Autodesk Inventor part; units mm, degrees
ref_plane "Plan de construction1" through (50, 0, -25) normal (0, 0, 1) x (1, 0, 0)
ref_plane "Plan de construction2" through (50, 0, 35) normal (0, 0, -1) x (-1, 0, 0)
ref_plane "YZ Plane" through (0, 0, 0) normal (1, 0, 0) x (0, 1, 0)
sketch "Esquisse1" plane through (0, 0, 0) normal (0, 1, 0) x (-1, 0, 0)
  line L0 (0, 0) -> (-100, 0)
  line L1 (-100, 0) -> (-100, -25)
  line L2 (-100, -25) -> (0, -25)
  line L3 (0, -25) -> (0, 0)
  arc A0 (0, -25) -> (25, 0) centre (0, 0) ccw
  line L4 (25, 0) -> (0, 0)
  line L5 (0, 0) -> (0, -25)
  line L6 (-100, 0) -> (-100, -25)
  arc A1 (-125, 0) -> (-100, -25) centre (-100, 0) ccw
  line L7 (-100, 0) -> (-125, 0)
  dimension "d1" = 25
  dimension "d2" = 100
revolve "Révolution1" add sketch "Esquisse1" angle 360 about axis through (0, 0, 0) along (1, 0, 0)
ref_plane "Plan de construction1" through (50, 0, -25) normal (0, 0, 1) x (1, 0, 0)
sketch "Esquisse2" plane through (50, 0, -25) normal (0, 0, 1) x (1, 0, 0)
  arc A0 (-50, 25) -> (-50, -25) centre (-50, 0) ccw
  line L0 (-50, 0) -> (-71.6506, -12.5)
  line L1 (-71.6506, -12.5) -> (-84.1506, 9.1506)
  line L2 (-84.1506, 9.1506) -> (-62.5, 21.6506)
  line L3 (-62.5, 21.6506) -> (-50, 0)
  line L4 (-50, 0) -> (-31.3481, 0) construction
  line L5 (-50, 0) -> (-62.5, 21.6506)
  line L6 (-62.5, 21.6506) -> (-19.1987, 46.6506)
  line L7 (-19.1987, 46.6506) -> (-6.6987, 25)
  line L8 (-6.6987, 25) -> (-50, 0)
  line L9 (-50, -25) -> (-50, 25) construction
  line L10 (-50, 25) -> (75, 25) construction
  line L11 (-50, 25) -> (50, 25) construction
  dimension "d9" = 120
extrude "Extrusion1" cut sketch "Esquisse2" along normal blind 30
ref_plane "Plan de construction2" through (50, 0, 35) normal (0, 0, -1) x (-1, 0, 0)
sketch "Esquisse3" plane through (50, 0, 35) normal (0, 0, -1) x (-1, 0, 0)
  line L0 (50, 0) -> (71.2132, -12.2474) construction
  line L1 (71.2132, -12.2474) -> (50, 0) construction
  line L2 (50, 0) -> (50, 0) construction
  line L3 (65.2228, 7.3769) -> (52.2324, 14.8769) construction
  circle A0 centre (65.2228, 7.3769) radius 1.7
  circle A1 centre (52.2324, 14.8769) radius 1.7
  line L4 (71.2132, -12.2474) -> (93.5005, 26.3552) construction
  line L5 (52.2324, 14.8769) -> (45.2324, 2.7526) construction
  line L6 (6.6987, 25) -> (-50, 25) construction
  dimension "d12" = 14
  dimension "d22" = 3.4
  dimension "d23" = 3.4
  dimension "d30" = 15
  dimension "d31" = 30
extrude "Extrusion2" cut sketch "Esquisse3" along normal blind 30
sketch "Esquisse4" plane through (50, 0, 35) normal (0, 0, -1) x (-1, 0, 0)
  circle A0 centre (65.2228, 7.3769) radius 1.7
  circle A1 centre (65.2228, 7.3769) radius 3.25
  circle A2 centre (52.2324, 14.8769) radius 1.7
  circle A3 centre (52.2324, 14.8769) radius 3.25
  point P0 (50, 0)
  dimension "d26" = 6.5
  dimension "d27" = 6.5
extrude "Extrusion3" cut sketch "Esquisse4" along normal blind 20
equation "\"d23\" = d22"
equation "\"d27\" = d26"
properties part number "P1704_003_mainGauche"
Check sheet for the modelled part. Datum: model origin and axes. Units: mm. A direction names the side the tool comes from. Round coordinates to 2 decimals unless told otherwise and drop trailing zeros. Loops run counter-clockwise (first coordinate to the right, second up) from the corner with the lowest first, then second, coordinate; pieces in that order, holes last. Notation, with made-up numbers: (-40, 48) - (-30, 48) arc R4 ccw to (-30, 52) - close; hole circle Ø10 at (65, 52.25). An arc over 180 degrees is marked (long way). Write item = value, one per line. Start each with the question number.
Q1. Section check A-A (x = 97). Record the boundary of the cut face in (y, z), plus the area to 3 significant figures.
Q2. Thickness scan on L1, parallel to Y at x = 0.5, z = 6; L2, parallel to X at y = 0, z = 7; L3, parallel to Z at x = 103.5, y = -13.5. Record the ranges inside material, lowest first.
Q3. Section check B-B (y = -7.5). Record the boundary of the cut face in (x, z).
Q4. Section check C-C (z = 0). Record the boundary of the cut face in (x, y).
Q5. Release check for a two-part mould opening along X. For faces 1 (the face through (1, 10, 5)), 2 (the face through (-16.793, 8.028, 10.07)) record: pulls with the +X half, pulls with the -X half, needs draft (parallel to the pull), parting line crosses it, or undercut.
Q6. Section check D-D (z = -12). Record the boundary of the cut face in (x, y).
Q7. Depth check by flat-ended pin: P1, Ø2, axis at x = -15.22, y = 7.38, coming from the -Z side; P2, Ø5, axis at x = -2.23, y = 14.88, coming from the -Z side; P3, Ø1, axis at x = 67.5, z = -19, coming from the +Y side; P4, Ø6, axis at x = 82.5, y = 11, coming from the -Z side. Enter the tip coordinate at first touch or a pass-through.
Q8. Access from +Z, -Z, +X, -X, +Y, -Y to the whole of each face (thin tool, end or side, straight path). Record for faces 3 (the face through (-0.88, 15.91, 10.07)), 4 (the face through (-12.356, 5.846, 17.349)).
Derived:
q1.outline = circle Ø50 at (0, 0)
q1.area = 1,960 mm^2
q2.L1 = -24.27 to 24.27
q2.L2 = -24 to 124
q2.L3 = -20.75 to 20.75
q3.outline = (-23.32, 5) - (-12.99, 5) - (-12.99, -20) arc R23.85 ccw to (0, -23.85) - (100, -23.85) arc R23.85 ccw to (100, 23.85) - (0, 23.85) arc R23.85 ccw to start
q4.outline = (-21.65, -12.5) arc R25 ccw to (0, -25) - (100, -25) arc R25 ccw to (100, 25) - (43.3, 25) - (0, 0) - close
q5.face_1 = needs draft
q5.face_2 = undercut
q6.outline = (-18.99, -10.97) arc R21.93 ccw to (0, -21.93) - (100, -21.93) arc R21.93 ccw to (100, 21.93) - (37.99, 21.93) - (0, 0) - close
q7.P1 = through
q7.P2 = 5
q7.P3 = 16.82
q7.P4 = -23.69
q8.face_3 = +Z, -Z
q8.face_4 = +Z
